Can you work these out from the model? Positions are in its coordinate system, mm. Give positions to 0.01 mm unless a question says otherwise; leave off trailing zeros. Order: outer loops, then holes, each group sorted by start corner. A loop starts at its lowest first (then second) coordinate and runs counter-clockwise, first axis right, second up. Notation, with made-up numbers: (-11, 74) - (40, 74) arc R16 ccw to (40, 105) - close; hole circle Ø11 at (62, 35). An arc over 180 degrees is marked (long way). Answer as a JSON object with one key per item and string values.
```python
from build123d import *

# Parameters (mm, degrees)
SKETCH1_W           = 26.67
SKETCH1_H           = 20.32
SKETCH1_R           = 1.45
BOSS_EXTRUDE1_DEPTH = 3
FILLET1_R           = 3


with BuildPart() as part:
    # Sketch1 → Boss-Extrude1 (new body)
    with BuildSketch(Plane(origin=(0, 0, 0), x_dir=(1, 0, 0), z_dir=(0, 1, 0))):
        Rectangle(SKETCH1_W, SKETCH1_H)
        with Locations((-10.795, 7.62)):
            Circle(SKETCH1_R, mode=Mode.SUBTRACT)
        with Locations((-10.795, -7.62)):
            Circle(SKETCH1_R, mode=Mode.SUBTRACT)
        with Locations((10.795, -7.62)):
            Circle(SKETCH1_R, mode=Mode.SUBTRACT)
        with Locations((10.795, 7.62)):
            Circle(SKETCH1_R, mode=Mode.SUBTRACT)
    extrude(amount=BOSS_EXTRUDE1_DEPTH)

    # Fillet1
    fillet1_edges = [part.edges().sort_by_distance(p)[0] for p in [
        (13.335, 1.5, 10.16),
        (-13.335, 1.5, 10.16),
        (-13.335, 1.5, -10.16),
        (13.335, 1.5, -10.16),
    ]]
    fillet(fillet1_edges, radius=FILLET1_R)


solid = part.part
```
Q1. We'd pull the mould along Z, two halves only. Please class faces 1 (the face through (0, 0, 0)), 2 (the face through (-9.456, 1.479, 8.175)), 3 (the face through (12.433, 1.521, 9.305)), 4 (the face through (12.433, 1.521, -9.305)): released by +Z, released by -Z, zero draft, split by the parting line, or undercut.
Recorded:
{"face 1": "zero draft", "face 2": "undercut", "face 3": "released by +Z", "face 4": "released by -Z"}
Q2. If we section it at C-C, the plane z = -7.62: Please give me the cut outline in (x, y) (3 decimals), then the cut area to 3 significant figures.
Recorded:
{"outline": "(-13.3, 0) - (-12.245, 0) - (-12.245, 3) - (-13.3, 3) - close; (-9.345, 0) - (9.345, 0) - (9.345, 3) - (-9.345, 3) - close; (12.245, 0) - (13.3, 0) - (13.3, 3) - (12.245, 3) - close", "area": "62.4 mm^2"}
Q3. I need wall thicknesses on L1, parallel to Z at x = -11.25, y = 2.25; L2, parallel to Z at x = 10.25, y = 2.15; L3, parallel to X at y = 1.6, z = -7.62 (3 decimals). Which ranges of each line are inside material? Lowest first, please.
Recorded:
{"L1": "z = -10.02 to -9, -6.24 to 6.24, 9 to 10.02", "L2": "z = -10.16 to -8.96, -6.28 to 6.28, 8.96 to 10.16", "L3": "x = -13.3 to -12.245, -9.345 to 9.345, 12.245 to 13.3"}
Q4. If we section it at B-B, the plane z = 6.75: Please give me the cut outline in (x, y) (3 decimals).
Recorded:
{"outline": "(-13.335, 0) - (-11.955, 0) - (-11.955, 3) - (-13.335, 3) - close; (-9.635, 0) - (9.635, 0) - (9.635, 3) - (-9.635, 3) - close; (11.955, 0) - (13.335, 0) - (13.335, 3) - (11.955, 3) - close"}
Q5. If we section it at A-A, the plane y = 0.3: Please give me the cut outline in (x, z) (3 decimals), then the cut area to 3 significant figures.
Recorded:
{"outline": "(-13.335, -7.16) arc R3 ccw to (-10.335, -10.16) - (10.335, -10.16) arc R3 ccw to (13.335, -7.16) - (13.335, 7.16) arc R3 ccw to (10.335, 10.16) - (-10.335, 10.16) arc R3 ccw to (-13.335, 7.16) - close; hole circle Ø2.9 at (-10.795, -7.62); hole circle Ø2.9 at (-10.795, 7.62); hole circle Ø2.9 at (10.795, -7.62); hole circle Ø2.9 at (10.795, 7.62)", "area": "508 mm^2"}
